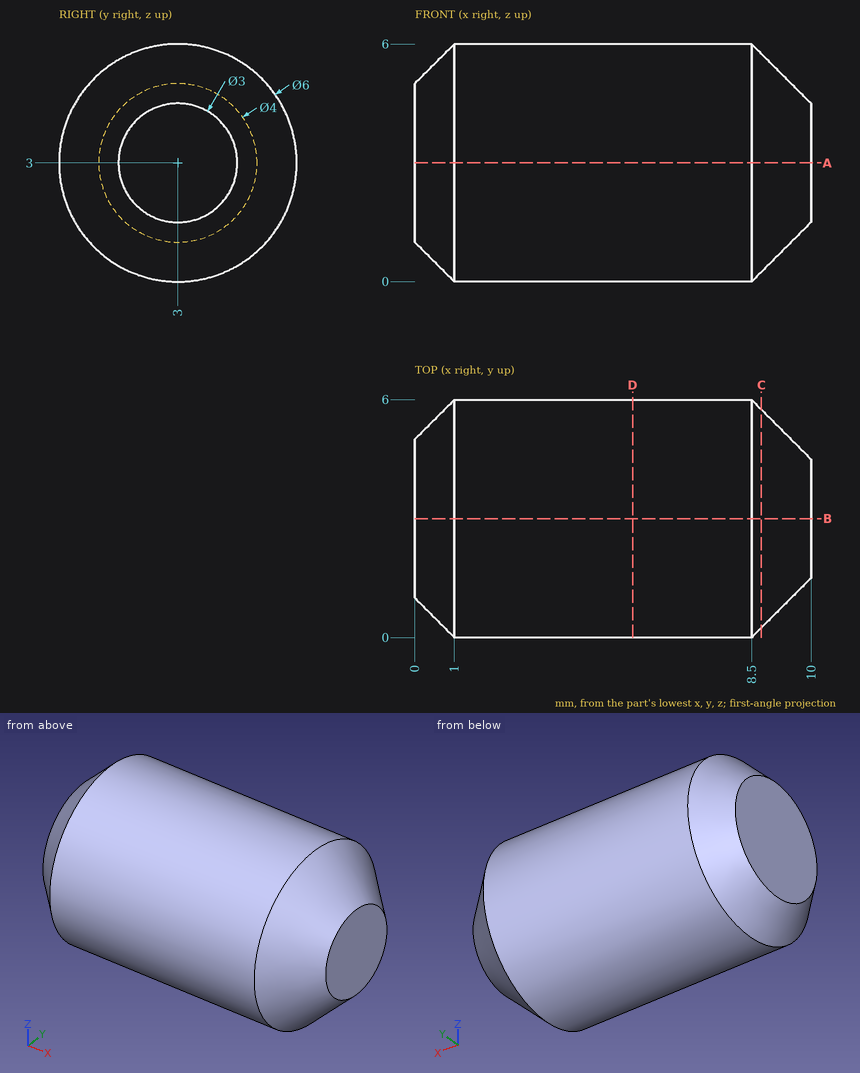
Geometry: see drawing. Coordinates: mm, zero at the bounding-box minimum. Give positions to 0.01 mm unless a question says otherwise; leave off trailing zeros. Order: outer loops, then holes, each group sorted by start corner. A loop starts at its lowest first (then second) coordinate and runs counter-clockwise, first axis right, second up. Notation, with made-up numbers: (63.25, 15) -> (70.25, 15) arc R8 ccw to (70.25, 25) -> close; hole circle Ø10 at (-37.5, 62.5). An arc over 180 degrees is marked (long way). Write each question's results on one line, items separated by ' | '.
1) Cut plane A-A (z = 3). Output: boundary loops of the cut face in (x, y).
Geometry says:
outline: (0, 1) -> (1, 0) -> (8.5, 0) -> (10, 1.5) -> (10, 4.5) -> (8.5, 6) -> (1, 6) -> (0, 5) -> close
2) Line query: line 1 along Z through (x, y) = (4.75, 1.1); line 2 along X through (y, z) = (0.75, 4.45); line 3 along X through (y, z) = (4.25, 2). Output: solid intervals per line, ascending.
Geometry says:
line 1: z = 0.68 to 5.32 | line 2: x = 0.68 to 8.82 | line 3: x = 0 to 9.9
3) Cut plane D-D (x = 5.5). Output: boundary loops of the cut face in (y, z), and give its area (3 significant figures).
Geometry says:
outline: circle Ø6 at (3, 3) | area: 28.3 mm²
4) Cut plane C-C (x = 8.75). Output: boundary loops of the cut face in (y, z).
Geometry says:
outline: circle Ø5.5 at (3, 3)
